```python
from build123d import *

# Parameters (mm, degrees)
SKETCH_1_R          = 1.25
SKETCH_1_W          = 25
SKETCH_1_H          = 11.6
EXTRUDE_2_DEPTH     = 4
EXTRUDE_3_DEPTH     = 12
SKETCH_2_R          = 1.5
CUT_EXTRUDE_1_DEPTH = 12.993


with BuildPart() as part:
    # Sketch 1 → Extrude 2 (new body)
    with BuildSketch(Plane.XY):
        with BuildLine():
            Line((41.271371981, 0), (18.571371981, 0))
            Line((18.571371981, 0), (15.754115944, 0))
            ThreePointArc((15.754115944, 0), (13.648249367, -0.465099124), (11.934157469, -1.773869616))
            Line((11.934157469, -1.773869616), (10.238822763, -3.781261572))
            Line((10.238822763, -3.781261572), (-2.059131374, -17.607))
            Line((-2.059131374, -17.607), (4.182743963, -17.607))
            Line((4.182743963, -17.607), (13.591371981, -17.607))
            Line((13.591371981, -17.607), (13.591371981, -29.6))
            Line((13.591371981, -29.6), (43.591371981, -29.6))
            Line((43.591371981, -29.6), (43.591371981, -17.607))
            Line((43.591371981, -17.607), (53, -17.607))
            Line((53, -17.607), (59.241875336, -17.607))
            Line((59.241875336, -17.607), (46.9439212, -3.781261572))
            Line((46.9439212, -3.781261572), (45.248586493, -1.773869616))
            ThreePointArc((45.248586493, -1.773869616), (43.534494596, -0.465099124), (41.428628019, 0))
            Line((41.428628019, 0), (41.271371981, 0))
        make_face()
        with Locations((13.591371981, -10.8)):
            Circle(SKETCH_1_R, mode=Mode.SUBTRACT)
        with Locations((28.771371981, -10.8)):
            Rectangle(SKETCH_1_W, SKETCH_1_H, mode=Mode.SUBTRACT)
        with Locations((43.591371981, -10.8)):
            Circle(SKETCH_1_R, mode=Mode.SUBTRACT)
    extrude(amount=EXTRUDE_2_DEPTH)

    # Sketch 1_4 → Extrude 3 (add)
    with BuildSketch(Plane.XY):
        with BuildLine():
            Line((13.591371981, -17.607), (-2.059131374, -17.607))
            ThreePointArc((-2.059131374, -17.607), (-2.621323899, -18.533838426), (-2.817256037, -19.6))
            Line((-2.817256037, -19.6), (-2.817256037, -26.6))
            ThreePointArc((-2.817256037, -26.6), (-1.938576381, -28.721320344), (0.182743963, -29.6))
            Line((0.182743963, -29.6), (13.591371981, -29.6))
            Line((13.591371981, -29.6), (13.591371981, -17.607))
        make_face()
        with BuildLine():
            ThreePointArc((60, -19.6), (59.804067862, -18.533838426), (59.241875336, -17.607))
            Line((59.241875336, -17.607), (43.591371981, -17.607))
            Line((43.591371981, -17.607), (43.591371981, -29.6))
            Line((43.591371981, -29.6), (57, -29.6))
            ThreePointArc((57, -29.6), (59.121320344, -28.721320344), (60, -26.6))
            Line((60, -26.6), (60, -19.6))
        make_face()
    extrude(amount=EXTRUDE_3_DEPTH)

    # Sketch 2 → Cut-Extrude 1 (cut, through all)
    with BuildSketch(Plane(origin=(0, -17.607, 0), x_dir=(1, 0, 0), z_dir=(0, 1, 0))):
        with Locations((2.591371981, -7.929255465)):
            Circle(SKETCH_2_R)
        with Locations((54.591371981, -7.929255465)):
            Circle(SKETCH_2_R)
    extrude(amount=-CUT_EXTRUDE_1_DEPTH, mode=Mode.SUBTRACT)


solid = part.part
```
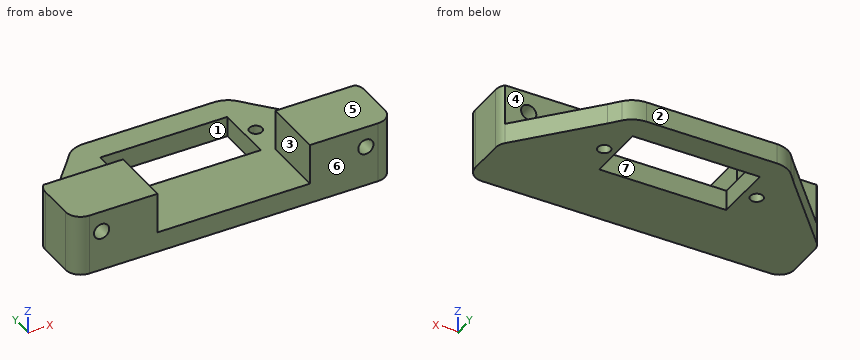
Input: part model. Units: mm. Frame: model coordinates. Face numbers are marked on the shaded views. A direction names the side the tool comes from. Coordinates: 2 decimals unless noted, no trailing zeros. Order: outer loops, then holes, each group sorted by start corner. A loop starts at its lowest first (then second) coordinate and runs counter-clockwise, first axis right, second up. Notation, with made-up numbers: (27, 7) - (34, 7) arc R33 ccw to (34, 37) - close; hole circle Ø9 at (39.25, 78.5). An arc over 180 degrees is marked (long way). Return JSON: item names as keys, results as strings.
Q1. First-contact query: pin 1 (6 mm diameter, centred on x = 4, z = 7.5, fed in from +Y); pin 2 (1 mm diameter, centred on x = 48, y = -13, fed in from +Z); pin 3 (4.5 mm diameter, centred on y = -10.5, z = 2, fed in from -X); pin 4 (5 mm diameter, centred on y = -17, z = 8.5, fed in from -X). Flat tips, straight axial feed; report the tip coordinate or a pass-through.
The answers:
{"pin 1": "stops at y = -17.61", "pin 2": "stops at z = 4", "pin 3": "stops at x = 2.26", "pin 4": "stops at x = -2.82"}
Q2. Access query for the marked faces 1, 2, 3 and 4. Directions: +Z, -Z, +X, -X, +Y, -Y. A direction counts if a zero-diameter tool reaches every point of the face in a straight line with its end or side. Return the directions, or none.
The answers:
{"face 1": "+Z, -Z", "face 2": "+Z, -Z, +X, -X, +Y", "face 3": "+Z, +Y, -Y", "face 4": "+Z, +X, -X, +Y"}
Q3. Cut plane C-C (y = -10.8). Return loops of the section in (x, z), then the cut area to 3 significant figures.
The answers:
{"outline": "(4, 0) - (12.34, 0) - (12.34, 4) - (4, 4) - close; (14.84, 0) - (16.27, 0) - (16.27, 4) - (14.84, 4) - close; (41.27, 0) - (42.34, 0) - (42.34, 4) - (41.27, 4) - close; (44.84, 0) - (53.19, 0) - (53.19, 4) - (44.84, 4) - close", "area": "76.8 mm2"}
Q4. Cut plane B-B (z = 10.5). Return loops of the section in (x, y).
The answers:
{"outline": "(-2.82, -26.6) arc R3 ccw to (0.18, -29.6) - (13.59, -29.6) - (13.59, -17.61) - (-2.06, -17.61) arc R3 ccw to (-2.82, -19.6) - close; (43.59, -29.6) - (57, -29.6) arc R3 ccw to (60, -26.6) - (60, -19.6) arc R3 ccw to (59.24, -17.61) - (43.59, -17.61) - close"}
Q5. Cut plane A-A (x = 40). Return loops of the section in (y, z).
The answers:
{"outline": "(-29.6, 0) - (-16.6, 0) - (-16.6, 4) - (-29.6, 4) - close; (-5, 0) - (0, 0) - (0, 4) - (-5, 4) - close"}
Q6. Draft query along Y for the marked faces 5, 6 and 7. Return one class per face: +Y half, -Y half, draft (parallel to the pull), parting line (faces both ways), or undercut.
The answers:
{"face 5": "draft", "face 6": "-Y half", "face 7": "undercut"}
Q7. Ray query, probe 1 along X at (y, z) = (-22.25, 6); probe 2 along Z at (x, y) = (43.5, -22.5); probe 3 along Y at (x, z) = (9, 9.75). Return the intervals inside material, ascending.
The answers:
{"probe 1": "x = -2.82 to 13.59, 43.59 to 60", "probe 2": "z = 0 to 4", "probe 3": "y = -29.6 to -17.61"}
Q8. Cut plane D-D (y = -24). Return loops of the section in (x, z).
The answers:
{"outline": "(-2.82, 0) - (60, 0) - (60, 12) - (43.59, 12) - (43.59, 4) - (13.59, 4) - (13.59, 12) - (-2.82, 12) - close; hole circle Ø3 at (2.59, 7.93); hole circle Ø3 at (54.59, 7.93)"}
